from build123d import *

# Parameters (mm, degrees)
SKETCH1_W           = 24
SKETCH1_H           = 12
BOSS_EXTRUDE1_DEPTH = 1
SKETCH2_W           = 12
SKETCH2_H           = 50.87
BOSS_EXTRUDE2_DEPTH = 2
BOSS_EXTRUDE3_DEPTH = 1.5
SKETCH5_W           = 12
SKETCH5_H           = 4
BOSS_EXTRUDE4_DEPTH = 2


with BuildPart() as part:
    # Sketch1 → Boss-Extrude1 (new, symmetric)
    with BuildSketch(Plane(origin=(0, 0, 0), x_dir=(1, 0, 0), z_dir=(0, 1, 0))):
        Rectangle(SKETCH1_W, SKETCH1_H)
    extrude(amount=BOSS_EXTRUDE1_DEPTH, both=True)

    # Sketch2 → Boss-Extrude2 (add)
    with BuildSketch(Plane.ZY.offset(12)):
        with Locations((0, -24.435)):
            Rectangle(SKETCH2_W, SKETCH2_H)
    boss_extrude2 = extrude(amount=BOSS_EXTRUDE2_DEPTH)

    # Mirror1: Boss-Extrude2 across plane
    add(boss_extrude2.mirror(Plane(origin=(0, 0, 0), x_dir=(0, 0, 1), z_dir=(1, 0, 0))))

    # Sketch4 → Boss-Extrude3 (add)
    with BuildSketch(Plane(origin=(-12, 0, 0), x_dir=(0, 0, -1), z_dir=(1, 0, 0))):
        with BuildLine():
            Line((-6, -47.300004682), (-6, -49.87))
            Line((-6, -49.87), (6, -49.87))
            Line((6, -49.87), (6, -47.300004682))
            ThreePointArc((6, -47.300004682), (0, -48.87), (-6, -47.300004682))
        make_face()
    extrude(amount=BOSS_EXTRUDE3_DEPTH)

    # Sketch5 → Boss-Extrude4 (add)
    with BuildSketch(Plane(origin=(-10.5, 0, 0), x_dir=(0, 0, -1), z_dir=(1, 0, 0))):
        with Locations((0, -47.87)):
            Rectangle(SKETCH5_W, SKETCH5_H)
    extrude(amount=BOSS_EXTRUDE4_DEPTH)


solid = part.part
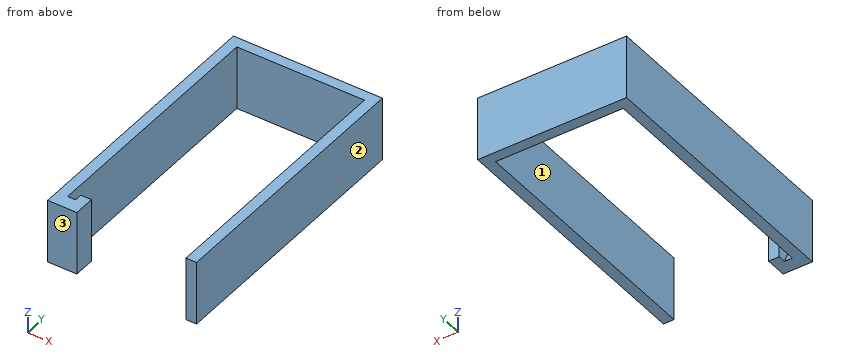
Source: CAD feature listing. Evaluate the final solid. Frame: model axes, mm. Face numbers are marked on the shaded views. Round coordinates to 2 decimals unless told otherwise and drop trailing zeros. Loops run counter-clockwise (first coordinate to the right, second up) from the corner with the lowest first, then second, coordinate; pieces in that order, holes last. Notation, with made-up numbers: M 41.5,76.25 L 65.5,76.25 A22 ccw 65.5,85.25 Z; hole C -10,73 d5. An arc over 180 degrees is marked long. Return JSON: item names as keys, results as strings. Group by question number.
1. Material intervals for line 1 along X through (y, z) = (-27.5, -1.25); line 2 along X through (y, z) = (-48, -4.25); line 3 along Y through (x, z) = (-10.25, -5), sorted ascending. Write a range as from..to.
2. Pin query (flat end, axial travel): pin 1 (1.5 mm diameter, centred on x = 9.5, y = -38.5, fed in from +Z); pin 2 (3.5 mm diameter, centred on x = 2, z = -2.5, fed in from -Y); pin 3 (1.5 mm diameter, centred on x = -8, z = 3, fed in from -Y). Return the tip coordinate at first contact, or that it passes through.
3. Section query B-B on x = -11. Output: boundary loops of the cut face in (y, z), and give its area (3 significant figures).
4. Section query D-D on x = 7. Output: boundary loops of the cut face in (y, z), and give its area (3 significant figures).
5. Section query A-A on y = -28. Output: boundary loops of the cut face in (x, z).
6. Mould query, pull axis X, two halves, no side actions, for the marked faces 1, 2 and 3. Classes: released by +X, released by -X, zero draft, split by the parting line, or undercut.
7. Section query C-C on z = -1. Output: boundary loops of the cut face in (x, y).
Checks:
{
 "1": {"line 1": "x = -14..-12, 12..14", "line 2": "x = -14..-12, -10.5..-8.5, 12..14", "line 3": "y = -49.87..-45.87, -1..1"},
 "2": {"pin 1": "passes through", "pin 2": "stops at y = -1", "pin 3": "stops at y = -49.87"},
 "3": {"outline": "M -49.87,-6 L -47.3,-6 A12.25 cw -47.3,6 L -49.87,6 Z; M -1,-6 L 1,-6 L 1,6 L -1,6 Z", "area": "42.1 mm²"},
 "4": {"outline": "M -1,-6 L 1,-6 L 1,6 L -1,6 Z", "area": "24.0 mm²"},
 "5": {"outline": "M -14,-6 L -12,-6 L -12,6 L -14,6 Z; M 12,-6 L 14,-6 L 14,6 L 12,6 Z"},
 "6": {"face 1": "undercut", "face 2": "released by +X", "face 3": "zero draft"},
 "7": {"outline": "M -14,-49.87 L -8.5,-49.87 L -8.5,-45.87 L -10.5,-45.87 L -10.5,-48.83 L -12,-48.83 L -12,-1 L 12,-1 L 12,-49.87 L 14,-49.87 L 14,1 L -14,1 Z"}
}
